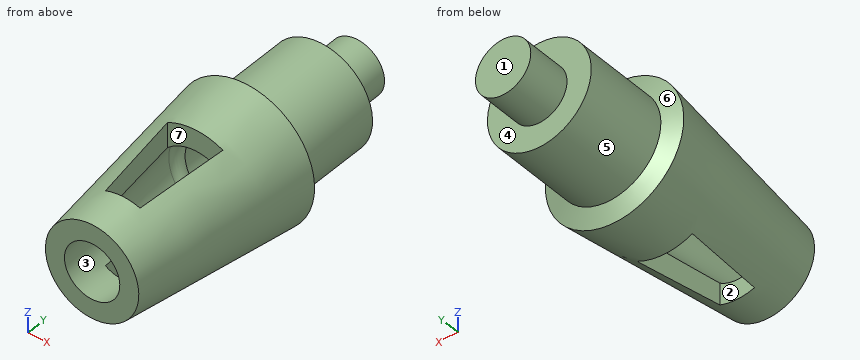
```python
from build123d import *

# Parameters (mm, degrees)
CUT_EXTRUDE1_DEPTH      = 199.242276016
CUT_EXTRUDE1_DEPTH_BACK = 199.242276016


with BuildPart() as part:
    # Sketch1 → Revolve1 (revolve)
    with BuildSketch(Plane.XY, mode=Mode.PRIVATE) as revolve1_sk:
        with BuildLine():
            Line((16, 0), (27, 0))
            Line((27, 0), (40, 110))
            Line((40, 110), (30, 114))
            Line((30, 114), (30, 164))
            Line((30, 164), (16, 164))
            Line((16, 164), (16, 190))
            Line((16, 190), (0, 190))
            Line((0, 190), (0, 147.51886968))
            Line((0, 147.51886968), (20, 147.51886968))
            Line((20, 147.51886968), (20, 91.51886968))
            ThreePointArc((20, 91.51886968), (23.714454765, 89.865931944), (24.97300455, 86))
            Line((24.97300455, 86), (16, 0))
        make_face()
    revolve(revolve1_sk.sketch.rotate(Axis((0, 273.925007331, 0), (0, -1, 0)), 90), axis=Axis((0, 273.925007331, 0), (0, -1, 0)))

    # Sketch2 → Cut-Extrude1 (cut, two sides: drawn at the far end of the back side and taken through both)
    with BuildSketch(Plane.XY.offset(-CUT_EXTRUDE1_DEPTH_BACK)):
        Polygon((-10, 22), (10, 22), (16, 74), (-16, 74), align=None)
    extrude(amount=CUT_EXTRUDE1_DEPTH + CUT_EXTRUDE1_DEPTH_BACK, mode=Mode.SUBTRACT)


solid = part.part
```
The listing builds one solid part. Answer for the finished solid, in the listing's coordinates (mm). Face numbers are marked on the shaded views. A direction names the side the tool comes from. Coordinates: 2 decimals unless noted, no trailing zeros. Write each loop counter-clockwise with the first axis right and the second up, starting at its lowest first coordinate (ties: lowest second). Pieces come first, ordered by that corner, then holes. Notation, with made-up numbers: (74.25, 2.5) - (131.25, 2.5) arc R19 cw to (131.25, 15.5) - close; hole circle Ø11 at (-4, -34). An arc over 180 degrees is marked (long way). One line per item, written item: value.
1) Consider line 1 along X through (y, z) = (132, 0); line 2 along Y through (x, z) = (0, 10.5); line 3 along X through (y, z) = (38.5, -19). Determine where each line is inside the solid, lowest interval first. Write a range as from..to.
Geometry check:
line 1: x = -30..-20, 20..30
line 2: y = 147.52..190
line 3: x = -25.19..-11.9, 11.9..25.19
2) Each of these flat-tipped pins is pushed along its axis until it touches: pin 1 Ø1.5 at (x, y) = (-25.5, 123.5) entering from +Z; pin 2 Ø4.5 at (x, z) = (4.5, 22) entering from +Y; pin 3 Ø2 at (x, y) = (-11, 25.5) entering from +Z. Where does it stop, or does it pass through?
Geometry check:
pin 1: stops at z = 16.95
pin 2: stops at y = 164
pin 3: stops at z = 28.23
3) A tool of negligible diameter and unlimited length cuts with its end or side. For the marked faces 1, 2, 3 and 4, from which of +Z, -Z, +X, -X, +Y, -Y can it reach the whole face along a straight path? Write none if from no direction.
Geometry check:
face 1: +Z, -Z, +X, -X, +Y
face 2: +Z, -Z
face 3: none
face 4: +Y
4) Find section D-D (y = 168.5). Give the vertices of the cut face in (x, z).
Geometry check:
outline: circle Ø32 at (0, 0)
5) Find section B-B (y = 137). Give the vertices of the cut face in (x, z), and give its area (3 significant figures).
Geometry check:
outline: circle Ø60 at (0, 0); hole circle Ø40 at (0, 0)
area: 1,570 mm2
6) For a pull along Y with two mould halves and no side action, classify the marked faces 5, 6 and 7 as pulls with the +Y half, pulls with the -Y half, needs draft (parallel to the pull), parting line crosses it, or undercut.
Geometry check:
face 5: needs draft
face 6: pulls with the +Y half
face 7: undercut
7) Find section A-A (z = 0). Give the vertices of the cut face in (x, y).
Geometry check:
outline: (-40, 110) - (-27, 0) - (-16, 0) - (-24.97, 86) arc R5 cw to (-20, 91.52) - (-20, 147.52) - (20, 147.52) - (20, 91.52) arc R5 cw to (24.97, 86) - (16, 0) - (27, 0) - (40, 110) - (30, 114) - (30, 164) - (16, 164) - (16, 190) - (-16, 190) - (-16, 164) - (-30, 164) - (-30, 114) - close
8) Find section C-C (x = 0). Give the vertices of the cut face in (y, z), and give its area (3 significant figures).
Geometry check:
outline: (0, -27) - (22, -29.6) - (22, -18.3) - (0, -16) - close; (0, 16) - (22, 18.3) - (22, 29.6) - (0, 27) - close; (74, -35.75) - (110, -40) - (114, -30) - (164, -30) - (164, -16) - (190, -16) - (190, 16) - (164, 16) - (164, 30) - (114, 30) - (110, 40) - (74, 35.75) - (74, 23.72) - (86, 24.97) arc R5 cw to (91.52, 20) - (147.52, 20) - (147.52, -20) - (91.52, -20) arc R5 cw to (86, -24.97) - (74, -23.72) - close
area: 4,240 mm2
